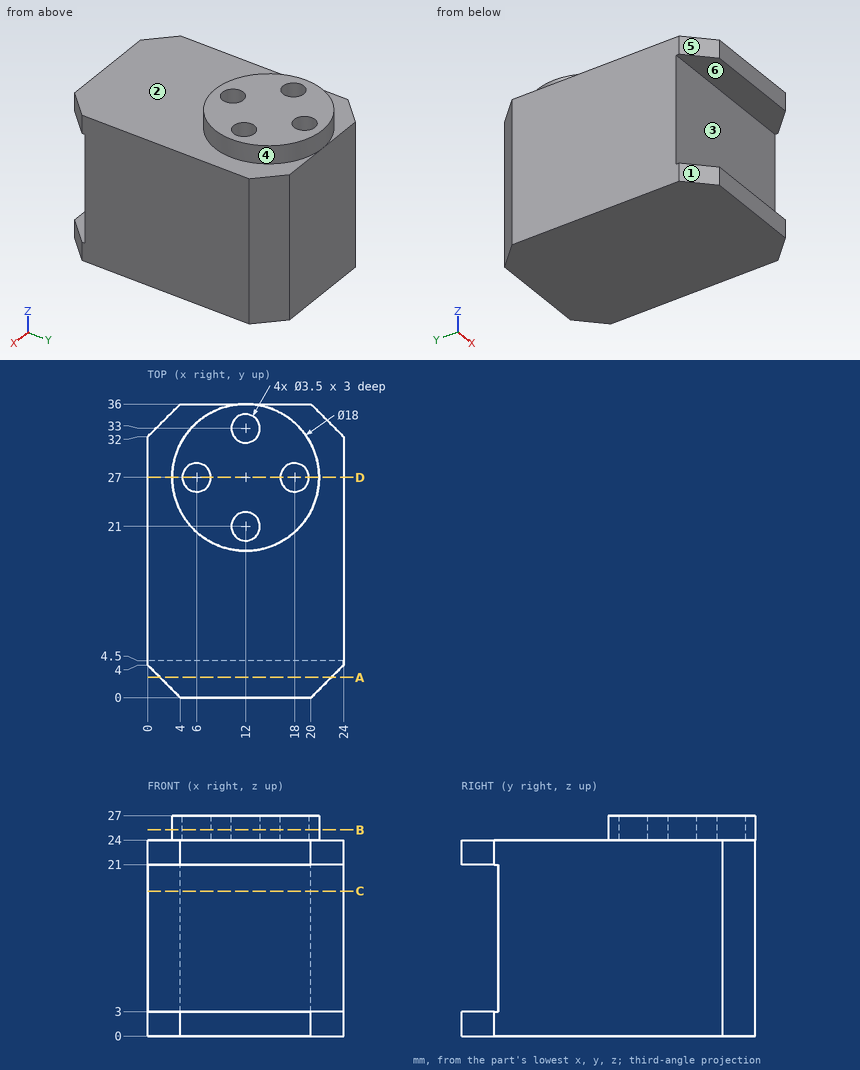
Print and shaded views of the part. All mm, measured from the part's lowest x, y and z. A direction names the side the tool comes from. Coordinates: 2 decimals unless noted, no trailing zeros. Loops run counter-clockwise (first coordinate to the right, second up) from the corner with the lowest first, then second, coordinate; pieces in that order, holes last. Notation, with made-up numbers: (33, 76.5) - (92, 76.5) arc R9 ccw to (92, 91.5) - close; hole circle Ø5 at (56.5, 38). An arc over 180 degrees is marked (long way). Write item = value, one per line. Start each with the question number.
Item 1: Drop flat-ended pins along their axis: pin 1 Ø12 at (x, z) = (6, 14) entering from -Y; pin 2 Ø1.8 at (x, y) = (11.5, 21.5) entering from +Z. Give the stop position or say it passes through.
Item 2: Saw through at B-B, the plane z = 25.25. List the corners of the cut face in (x, y).
Item 3: Pull direction Z, two halves, no side cores. Call the marked faces 1, 2 and 3: +Z half, -Z half, draft (parallel to the pull), parting line (faces both ways), or undercut.
Item 4: Wall check: probe 1 along X at (y, z) = (27, 25.8); probe 2 along Y at (x, z) = (13, 25.75); probe 3 along Z at (x, y) = (7.25, 4). Give the ranges that are in metal, low to high. Write a range as [from, to].
Item 5: Saw through at C-C, the plane z = 17.75. List the corners of the cut face in (x, y), then the cut area to 3 significant figures.
Item 6: 3-axis set-ups, long thin cutter, end or side, ignore diameter. For the marked faces 4, 5 and 6: which of +Z, -Z, +X, -X, +Y, -Y reach the whole face in a straight line?
Item 7: Saw through at D-D, the plane y = 27. List the corners of the cut face in (x, z), then the cut area to 3 significant figures.
Item 8: Saw through at A-A, the plane y = 2.5. List the corners of the cut face in (x, z), then the cut area to 3 significant figures.
Answers:
q1.pin_1 = 4.5
q1.pin_2 = 24
q2.outline = circle Ø18 at (12, 27); hole circle Ø3.5 at (6, 27); hole circle Ø3.5 at (12, 21); hole circle Ø3.5 at (12, 33); hole circle Ø3.5 at (18, 27)
q3.face_1 = draft
q3.face_2 = +Z half
q3.face_3 = undercut
q4.probe_1 = [3, 4.25], [7.75, 16.25], [19.75, 21]
q4.probe_2 = [18.06, 19.56], [22.44, 31.56], [34.44, 35.94]
q4.probe_3 = [0, 3], [21, 24]
q5.outline = (0, 4.5) - (24, 4.5) - (24, 32) - (20, 36) - (4, 36) - (0, 32) - close
q5.area = 740 mm2
q6.face_4 = +Z
q6.face_5 = +Z, -Z, -X, -Y
q6.face_6 = +X, -X, -Y
q7.outline = (0, 0) - (24, 0) - (24, 24) - (21, 24) - (21, 27) - (19.75, 27) - (19.75, 24) - (16.25, 24) - (16.25, 27) - (7.75, 27) - (7.75, 24) - (4.25, 24) - (4.25, 27) - (3, 27) - (3, 24) - (0, 24) - close
q7.area = 609 mm2
q8.outline = (1.5, 0) - (22.5, 0) - (22.5, 3) - (1.5, 3) - close; (1.5, 21) - (22.5, 21) - (22.5, 24) - (1.5, 24) - close
q8.area = 126 mm2
